Work out the finished part from the listing and answer in its coordinate system (mm). Face numbers are marked on the shaded views. A direction names the side the tool comes from. Give positions to 0.01 mm unless a question says otherwise; leave off trailing zeros. Write each loop counter-clockwise with the first axis right and the second up, starting at its lowest first coordinate (ties: lowest second). Pieces come first, ordered by that corner, then holes. Notation, with made-up numbers: (-4, 55.25) -> (48, 55.25) arc R24 ccw to (48, 90.25) -> close; hole circle Ø4 at (-25, 52). An arc over 180 degrees is marked (long way). Use a Markdown table: item, result. Add a question column.
Q1. Section A-A, the plane y = -12.7 is taken. Give the vertices of the cut face in (x, z) (1 decimal), plus the area to 3 significant figures.
Q2. For the marked faces 1, 2 and 3, determine the directions among +Z, -Z, +X, -X, +Y, -Y from which every point of the face is accessible in a straight line to the end or side of a thin tool.
Q3. Each of these flat-tipped pins is pushed along its axis until it touches: pin 1 Ø6 at (y, z) = (-18, -17.5) entering from -X; pin 2 Ø10 at (y, z) = (12.5, 3.5) entering from +X; pin 3 Ø8 at (y, z) = (2, -27) entering from -X. Where does it stop, or does it pass through?
Q4. Consider line 1 (X direction, y = -12, z = 7); line 2 (Z direction, x = 83, y = 10.5); line 3 (Y direction, x = 18, z = 7.5). Determine where each line is inside the solid, lowest interval first.
Q5. Section B-B, the plane x = 70 is taken. Give the vertices of the cut face in (y, z), plus the area to 3 significant figures.
Q6. For a pull along X with two mould halves and no side action, classify the marked faces 4, 5 and 6 as pulls with the +X half, pulls with the -X half, needs draft (parallel to the pull), parting line crosses it, or undercut.
Q7. Section C-C, the plane y = 1.5 is taken. Give the vertices of the cut face in (x, z), plus the area to 3 significant figures.
Q8. Section D-D, the plane z = -21 is taken. Give the vertices of the cut face in (x, y), plus the area to 3 significant figures.
from build123d import *

# Parameters (mm, degrees)
F1_DEPTH = 25.4
F3_DEPTH = 134.5312752574
F5_DEPTH = 118.5292752574
F6_R     = 3.9624
F7_DEPTH = 58.5522699094


with BuildPart() as f1:
    # F0 (on Front) → F1 (new body, symmetric)
    with BuildSketch(Plane.XZ):
        Polygon((0, 12.7), (0, 0), (85.852, 0), (131.7032699094, -45.8512699094), (149.6637821515, -27.8907576672), (111.5874961982, 10.1855282861), (102.6072400771, 1.205272165), (91.1125122421, 12.7), align=None)
    extrude(amount=F1_DEPTH, both=True)

    # F2 (on face) → F3 (cut, through all)
    with BuildSketch(Plane(origin=(88.7772699094, 0, -88.7772699094), x_dir=(0, 1, 0), z_dir=(0.7071067812, 0, -0.7071067812))):
        Polygon((9.652, 86.1065313784), (-9.652, 86.1065313784), (-9.652, 80.0105313784), (-15.748, 80.0105313784), (-15.748, 73.4065313784), (15.748, 73.4065313784), (15.748, 80.0105313784), (9.652, 80.0105313784), align=None)
    extrude(amount=-F3_DEPTH, mode=Mode.SUBTRACT)

    # F4 (on face) → F5 (cut, through all)
    with BuildSketch(Plane(origin=(60.8865122421, 0, 60.8865122421), x_dir=(0.7071067812, 0, -0.7071067812), z_dir=(0.7071067812, 0, 0.7071067812))):
        with BuildLine():
            ThreePointArc((119.183037491, 25.4), (125.5500191363, 0), (119.183037491, -25.4))
            Line((119.183037491, -25.4), (119.183037491, -33.2152206612))
            Line((119.183037491, -33.2152206612), (139.840820311, -33.2152206612))
            Line((139.840820311, -33.2152206612), (139.840820311, 34.853566438))
            Line((139.840820311, 34.853566438), (119.183037491, 34.853566438))
            Line((119.183037491, 34.853566438), (119.183037491, 25.4))
        make_face()
    extrude(amount=-F5_DEPTH, mode=Mode.SUBTRACT)

    # F6 (on face) → F7 (cut, through all)
    with BuildSketch(Plane.XY.offset(12.7)):
        with Locations((15.748, 12.7)):
            Circle(F6_R)
        with Locations((15.748, -12.7)):
            Circle(F6_R)
        with Locations((69.596, -12.7)):
            Circle(F6_R)
        with Locations((69.596, 12.7)):
            Circle(F6_R)
    extrude(amount=-F7_DEPTH, mode=Mode.SUBTRACT)


solid = f1.part
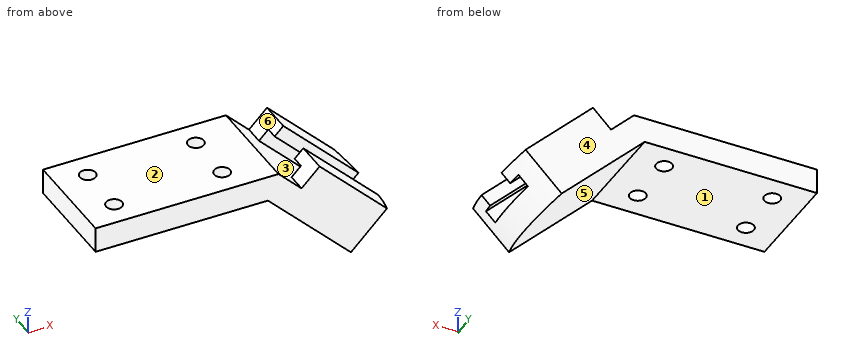
Result set:
| question | item | result |
|---|---|---|
| 1 | outline | (0, 0) -> (11.8, 0) -> (11.8, 12.7) -> (0, 12.7) -> close; (19.7, 0) -> (65.6, 0) -> (65.6, 12.7) -> (19.7, 12.7) -> close; (73.6, 0) -> (85.9, 0) -> (130.6, -44.8) -> (139.6, -35.8) -> (91.1, 12.7) -> (73.6, 12.7) -> close; (107.3, 5.9) -> (144.3, -31.1) -> (148.6, -26.8) -> (111.6, 10.2) -> close |
| 1 | area | 2,080 mm2 |
| 2 | face 1 | -Z, -X, +Y, -Y |
| 2 | face 2 | +Z, +X, -X, +Y, -Y |
| 2 | face 3 | none |
| 3 | pin 1 | stops at x = 100.35 |
| 3 | pin 2 | stops at x = 123.27 |
| 3 | pin 3 | stops at x = 108.85 |
| 4 | line 1 | x = 0 to 11.85, 19.65 to 65.7, 73.5 to 96.81, 108.4 to 114.77 |
| 4 | line 2 | z = 0 to 12.7 |
| 4 | line 3 | y = -25.4 to -15.96, -9.44 to 9.44, 15.96 to 25.4 |
| 5 | outline | (-25.4, 0) -> (-16.64, 0) -> (-16.64, 12.7) -> (-25.4, 12.7) -> close; (-8.76, 0) -> (8.76, 0) -> (8.76, 12.7) -> (-8.76, 12.7) -> close; (16.64, 0) -> (25.4, 0) -> (25.4, 12.7) -> (16.64, 12.7) -> close |
| 5 | area | 445 mm2 |
| 6 | face 4 | needs draft |
| 6 | face 5 | pulls with the -X half |
| 6 | face 6 | undercut |
| 7 | outline | (0, 0) -> (85.85, 0) -> (131.69, -45.84) -> (140.67, -36.86) -> (91.11, 12.7) -> (0, 12.7) -> close |
| 7 | area | 1,980 mm2 |
| 8 | outline | (106.85, -25.4) -> (142.77, -25.4) -> (142.77, -9.65) -> (134.15, -9.65) -> (134.15, -15.75) -> (124.81, -15.75) -> (124.81, 15.75) -> (134.15, 15.75) -> (134.15, 9.65) -> (142.77, 9.65) -> (142.77, 25.4) -> (106.85, 25.4) -> close |
| 8 | area | 1,360 mm2 |
